The listing builds one solid part. Answer for the finished solid, in the listing's coordinates (mm). Face numbers are marked on the shaded views. A direction names the side the tool comes from. Round coordinates to 2 decimals unless told otherwise and drop trailing zeros. Order: outer loops, then holes, each group sorted by start corner. A loop starts at its lowest first (then second) coordinate and runs counter-clockwise, first axis right, second up. Notation, with made-up numbers: (-24.5, -38) -> (32.5, -38) arc R22 ccw to (32.5, -24) -> close; hole circle Ø10 at (53.5, 38). An arc over 180 degrees is marked (long way). Return JSON: item names as keys, results as strings. Group by question number.
(1) The part is cut by section D-D (z = 10). Determine the outline of the cut face in (x, y).
(2) The part is cut by section A-A (y = 0). Determine the outline of the cut face in (x, z).
(3) Which of the six approach directions +Z, -Z, +X, -X, +Y, -Y give full straight-line access (tool end or side, diameter ignored) to the marked faces 1 and 2?
(4) Consider line 1 (Y direction, x = 0, z = 4); line 2 (Y direction, x = 0, z = 19.5); line 3 (X direction, y = 0.5, z = 16). Determine where each line is inside the solid, lowest interval first. Write a range as [from, to].
(5) Determine the mould class of the marked faces 3, 4 and 5 for opening direction X: +X half, -X half, draft (parallel to the pull), parting line (faces both ways), or undercut.
(6) The part is cut by section C-C (z = 21.25). Determine the outline of the cut face in (x, y).
(7) Each of these flat-tipped pins is pushed along its axis until it touches: pin 1 (1.5 mm diameter, centred on x = -5, y = 0.5, fed in from -Z); pin 2 (6 mm diameter, centred on x = -4, z = 15, fed in from +Y); pin 3 (2 mm diameter, centred on y = -3, z = 10.5, fed in from -X); pin 4 (1 mm diameter, centred on x = 0.5, y = 2.5, fed in from +Z). Where does it stop, or does it pass through?
from build123d import *

# Parameters (mm, degrees)
SKETCH1_R           = 7
BOSS_EXTRUDE1_DEPTH = 25
SKETCH3_R           = 4
CUT_EXTRUDE1_DEPTH  = 12.5
SKETCH4_R           = 2.5
CUT_EXTRUDE2_DEPTH  = 14.5
CHAMFER1_SIZE       = 0.5


with BuildPart() as part:
    # Sketch1 → Boss-Extrude1 (new body)
    with BuildSketch(Plane.XY):
        Circle(SKETCH1_R)
    extrude(amount=BOSS_EXTRUDE1_DEPTH)

    # Sketch3 → Cut-Extrude1 (cut)
    with BuildSketch(Plane.XY.offset(25)):
        Circle(SKETCH3_R)
    extrude(amount=-CUT_EXTRUDE1_DEPTH, mode=Mode.SUBTRACT)

    # Sketch4 → Cut-Extrude2 (cut)
    with BuildSketch(Plane.XY.offset(12.5)):
        Circle(SKETCH4_R)
    extrude(amount=-CUT_EXTRUDE2_DEPTH, mode=Mode.SUBTRACT)

    # Chamfer1
    chamfer1_edges = [part.edges().sort_by_distance(p)[0] for p in [
        (-7, 0, 0),
        (-7, 0, 25),
    ]]
    chamfer(chamfer1_edges, length=CHAMFER1_SIZE)


solid = part.part
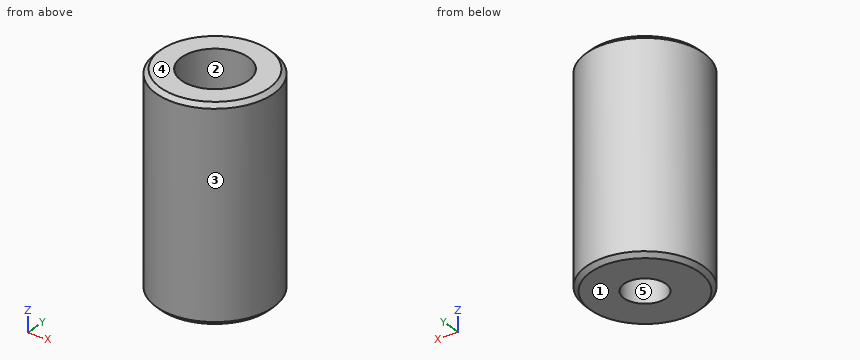
Answer below:
{
 "1": {"outline": "circle Ø14 at (0, 0); hole circle Ø5 at (0, 0)"},
 "2": {"outline": "(-7, 0.5) -> (-6.5, 0) -> (-2.5, 0) -> (-2.5, 12.5) -> (-4, 12.5) -> (-4, 25) -> (-6.5, 25) -> (-7, 24.5) -> close; (2.5, 0) -> (6.5, 0) -> (7, 0.5) -> (7, 24.5) -> (6.5, 25) -> (4, 25) -> (4, 12.5) -> (2.5, 12.5) -> close"},
 "3": {"face 1": "-Z, +X, -X, +Y, -Y", "face 2": "+Z"},
 "4": {"line 1": "y = [-7, -2.5], [2.5, 7]", "line 2": "y = [-7, -4], [4, 7]", "line 3": "x = [-6.98, -3.97], [3.97, 6.98]"},
 "5": {"face 3": "parting line", "face 4": "draft", "face 5": "undercut"},
 "6": {"outline": "circle Ø14 at (0, 0); hole circle Ø8 at (0, 0)"},
 "7": {"pin 1": "stops at z = 0", "pin 2": "stops at y = 6.93", "pin 3": "stops at x = -6.71", "pin 4": "stops at z = 12.5"}
}
